Verification items for the finished model (mm, model axes). Face numbers are marked on the shaded views. A direction names the side the tool comes from. Round coordinates to 2 decimals unless told otherwise and drop trailing zeros. Loops run counter-clockwise (first coordinate to the right, second up) from the corner with the lowest first, then second, coordinate; pieces in that order, holes last. Notation, with made-up numbers: (26, -30.75) -> (84, -30.75) arc R28 cw to (84, 6.25) -> close; hole circle Ø1 at (-18.5, 64). An arc over 180 degrees is marked (long way). Use a Markdown table: item, result. Add a question column.
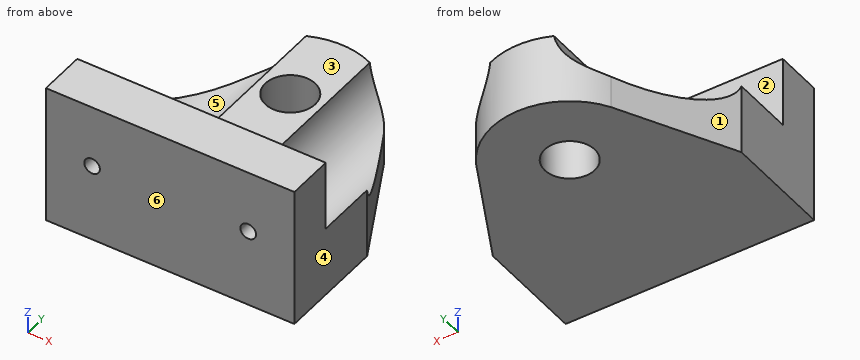
Autodesk Inventor part; units mm, degrees
ref_plane "YZ Plane" through (0, 0, 0) normal (1, 0, 0) x (0, 1, 0)
ref_plane "XZ Plane" through (0, 0, 0) normal (0, 1, 0) x (-1, 0, 0)
ref_plane "XY Plane" through (0, 0, 0) normal (0, 0, 1) x (1, 0, 0)
sketch "Sketch1" plane through (0, 0, 0) normal (0, 0, 1) x (1, 0, 0)
  circle A0 centre (10, 11.5) radius 1.6
  line L0 (0, 0) -> (20.0001, 0)
  line L1 (0, 0) -> (0, 3)
  line L2 (20.0001, 0) -> (20.0001, 3)
  line L3 (0, 3) -> (16, 3) construction
  line L4 (20.0001, 3) -> (36.0001, 3) construction
  arc A1 (14.3301, 14) -> (5.6699, 14) centre (10, 11.5) ccw
  line L5 (10, 11.5) -> (5.6699, 14) construction
  line L6 (10, 11.5) -> (14.3301, 14) construction
  line L7 (5.6699, 14) -> (0, 3)
  line L8 (14.3301, 14) -> (20.0001, 3)
  dimension "d17" = 3
  dimension "d18" = 3
  dimension "d19" = 11.5
  dimension "d23" = 90
  dimension "d24" = 90
  dimension "d25" = 10
  dimension "d31" = 5
  dimension "d32" = 120
  dimension "d33" = 14
extrude "Extrusion1" add sketch "Sketch1" along normal blind 4.5
sketch "Sketch4" plane through (0, 0, 4.5) normal (0, 0, 1) x (1, 0, 0)
  line L0 (0, 3) -> (0, 0)
  line L1 (20.0001, 0) -> (20.0001, 3)
  line L2 (0, 0) -> (20.0001, 0)
  line L3 (20.0001, 0) -> (20.0001, 3)
  line L4 (3.884, 22.9404) -> (-0.9789, 3.2417)
  line L5 (20.0001, 3) -> (0, 3)
  line L6 (0, 3) -> (0, 0)
extrude "Extrusion2" add sketch "Sketch4" along normal blind 4.5
sketch "Sketch5" plane through (0, 0, 0) normal (0, -1, 0) x (1, 0, 0)
  circle A0 centre (5, 5) radius 0.5
  circle A1 centre (15, 5) radius 0.5
  line L0 (0, 0) -> (20.0001, 0)
  dimension "d13" = 1
  dimension "d14" = 1
  dimension "d38" = 5
  dimension "d39" = 5
extrude "Extrusion3" cut sketch "Sketch5" against normal blind 5.5
sketch "Sketch6" plane through (0, 3, 9) normal (0, 1, 0) x (1, 0, 0)
  circle A0 centre (5, 4) radius 0.5
  circle A1 centre (5, 4) radius 3
  circle A2 centre (15, 4) radius 0.5
  circle A3 centre (15, 4) radius 3
  line L0 (0, 9) -> (20.0001, 9)
  dimension "d34" = 6
  dimension "d35" = 6
  dimension "d40" = 5
  dimension "d41" = 5
extrude "Extrusion4" cut sketch "Sketch6" along normal up to next
sketch "Sketch7" plane through (0, 0, 0) normal (0, -1, 0) x (1, 0, 0)
  line L0 (0, 0) -> (0, 9)
  line L1 (2.042, 0) -> (0, 0)
  line L2 (0, 0) -> (0, 9)
  line L3 (0, 9) -> (2.042, 9)
  line L4 (2.042, 9) -> (2.042, 0)
extrude "Extrusion5" cut sketch "Sketch7" against normal up to next
sketch "Sketch8" plane through (20.0001, 0, 0) normal (0, -1, 0) x (1, 0, 0)
  line L0 (0, 4.5) -> (0, 9)
  line L1 (-2.042, 0) -> (0, 0)
  line L2 (0, 0) -> (0, 9)
  line L3 (0, 9) -> (-2.042, 9)
  line L4 (-2.042, 9) -> (-2.042, 0)
  point P0 (-20.0001, 0)
extrude "Extrusion6" cut sketch "Sketch8" against normal up to next
properties part number "lower_deck_short_shaft_mount_for_AD"
1) Sectioned sample at C-C on z = 1. Enter the section's corners in (x, y).
2) Sectioned sample at B-B on x = 10. Enter the section's corners in (y, z).
3) Go/stop test with flat-tipped pins: pin 1 (3.5 mm diameter, centred on x = 9.5, y = 11, fed in from +Z); pin 2 (2 mm diameter, centred on x = 4, y = 7.5, fed in from +Z); pin 3 (1.5 mm diameter, centred on x = 7, z = 3, fed in from +Y). Record where each tip stops, or that it passes through.
4) Sectioned sample at A-A on z = 5. Enter the section's corners in (x, y).
5) Access from +Z, -Z, +X, -X, +Y, -Y to the whole of each face (thin tool, end or side, straight path). Record for the marked faces 1, 2 and 3.
6) Release check for a two-part mould opening along X. For the marked faces 4, 5 and 6 record: released by +X, released by -X, zero draft, split by the parting line, or undercut.
7) Thickness scan on line 1 (Z direction, x = 15, y = 0.95); line 2 (Y direction, x = 10, z = 2.95); line 3 (Y direction, x = 14, z = 4.25). Record the ranges inside material, lowest first.
8) Sectioned sample at D-D on y = 11.5. Enter the section's corners in (x, z).
Geometry results:
| question | item | result |
|---|---|---|
| 1 | outline | (2.04, 0) -> (17.96, 0) -> (17.96, 6.96) -> (14.33, 14) arc R5 ccw to (5.67, 14) -> (2.04, 6.96) -> close; hole circle Ø3.2 at (10, 11.5) |
| 2 | outline | (0, 0) -> (9.9, 0) -> (9.9, 4.5) -> (3, 4.5) -> (3, 9) -> (0, 9) -> close; (13.1, 0) -> (16.5, 0) -> (16.5, 4.5) -> (13.1, 4.5) -> close |
| 3 | pin 1 | z = 4.5 |
| 3 | pin 2 | z = 2.76 |
| 3 | pin 3 | y = 15.97 |
| 4 | outline | (2.04, 0) -> (4.5, 0) -> (4.5, 3) -> (2.04, 3) -> close; (5.5, 0) -> (14.5, 0) -> (14.5, 3) -> (5.5, 3) -> close; (15.5, 0) -> (17.96, 0) -> (17.96, 3) -> (15.5, 3) -> close |
| 5 | face 1 | +Z, -Z, -X, +Y |
| 5 | face 2 | +Z, +Y |
| 5 | face 3 | +Z, +X, -X, +Y |
| 6 | face 4 | released by +X |
| 6 | face 5 | undercut |
| 6 | face 6 | zero draft |
| 7 | line 1 | 0 to 4.5, 5.5 to 9 |
| 7 | line 2 | 0 to 9.9, 13.1 to 16.5 |
| 7 | line 3 | 0 to 3 |
| 8 | outline | (4.38, 0) -> (8.4, 0) -> (8.4, 4.5) -> (7.96, 4.5) arc R3 cw to (4.38, 2.06) -> close; (11.6, 0) -> (15.62, 0) -> (15.62, 2.06) arc R3 cw to (12.04, 4.5) -> (11.6, 4.5) -> close |
